Autodesk Inventor part; units mm, degrees
ref_plane "YZ Plane" through (0, 0, 0) normal (1, 0, 0) x (0, 1, 0)
ref_plane "XZ Plane" through (0, 0, 0) normal (0, 1, 0) x (-1, 0, 0)
ref_plane "XY Plane" through (0, 0, 0) normal (0, 0, 1) x (1, 0, 0)
sketch "Sketch1" plane through (0, 0, 0) normal (0, 0, 1) x (1, 0, 0)
  line L0 (-175.444, 104.3404) -> (240.5572, 104.3404)
  line L1 (240.5572, 104.3404) -> (240.5572, -311.6608)
  line L2 (113.5572, -311.6608) -> (-48.444, -311.6608)
  line L3 (-175.444, -311.6608) -> (-175.444, 104.3404)
  line L4 (-48.444, -311.6608) -> (-48.444, -343.6648)
  line L5 (-48.444, -343.6648) -> (-175.444, -343.6648)
  line L6 (-175.444, -343.6648) -> (-175.444, -311.6608)
  line L7 (113.5572, -311.6608) -> (113.5572, -343.6648)
  line L8 (113.5572, -343.6648) -> (240.5572, -343.6648)
  line L9 (240.5572, -343.6648) -> (240.5572, -311.6608)
  point P0 (0, 0)
  dimension "d0" = 416.0012
  dimension "d1" = 416.0012
  dimension "d2" = 127
  dimension "d3" = 127
  dimension "d4" = 162.0012
  dimension "d5" = 32.004
extrude "Extrusion1" add sketch "Sketch1" along normal blind 5.08
properties part number "plate"
Geometry check sheet. Reference: the model listing, model coordinates, mm. Give positions to 0.01 mm unless a question says otherwise; leave off trailing zeros. Write each loop counter-clockwise with the first axis right and the second up, starting at its lowest first coordinate (ties: lowest second). Pieces come first, ordered by that corner, then holes. Notation, with made-up numbers: (40.5, 74.25) - (72.5, 74.25) arc R24 ccw to (72.5, 89.25) - close; hole circle Ø11 at (44, -33.5). An arc over 180 degrees is marked (long way). Put each result on its own line as item: value.
1. Thickness scan on line 1 (X direction, y = -319, z = 2); line 2 (Y direction, x = 63.5, z = 0.8). Record the ranges inside material, lowest first.
Ans:
line 1: x = -175.44 to -48.44, 113.56 to 240.56
line 2: y = -311.66 to 104.34
2. Sectioned sample at B-B, the plane x = 34. Enter the section's corners in (y, z), plus the area to 3 significant figures.
Ans:
outline: (-311.66, 0) - (104.34, 0) - (104.34, 5.08) - (-311.66, 5.08) - close
area: 2,110 mm²
3. Go/stop test with a flat-tipped pin: pin 1 (2.5 mm diameter, centred on x = 55.5, z = 2, fed in from -Y). Record where the tip stops, or that it passes through.
Ans:
pin 1: stops at y = -311.66
4. Sectioned sample at A-A, the plane z = 1. Enter the section's corners in (x, y).
Ans:
outline: (-175.44, -343.66) - (-48.44, -343.66) - (-48.44, -311.66) - (113.56, -311.66) - (113.56, -343.66) - (240.56, -343.66) - (240.56, 104.34) - (-175.44, 104.34) - close
